Here's how the part is built. I have some questions about the finished solid (model axes, mm). A direction names the side the tool comes from. Give positions to 0.01 mm unless a question says otherwise; leave off trailing zeros. Loops run counter-clockwise (first coordinate to the right, second up) from the corner with the lowest first, then second, coordinate; pieces in that order, holes last. Notation, with made-up numbers: (57, 72.5) - (75, 72.5) arc R25 ccw to (75, 106.5) - close; hole circle Ø5 at (-12.5, 80). An arc over 180 degrees is marked (long way). Use one line per item in the form item = value.
from build123d import *

# Parameters (mm, degrees)
F0_W      = 139.7
F0_H      = 215.9
F1_DEPTH  = 74.7
F2_R      = 17.526
F2_R_2    = 14.351
F2_R_3    = 11.176
F3_DEPTH  = 0.5
F4_R      = 17.526
F4_R_2    = 14.351
F4_R_3    = 11.176
F5_DEPTH  = 1
F4_R_4    = 3.55
F6_DEPTH  = 25
F7_W      = 17.25
F7_H      = 1.4
F8_DEPTH  = 51.1
F10_DEPTH = 139.701
F11_R     = 2


with BuildPart() as f1:
    # F0 (on Right) → F1 (new body, symmetric)
    with BuildSketch(Plane.YZ):
        with Locations((69.85, 107.95)):
            Rectangle(F0_W, F0_H)
    extrude(amount=F1_DEPTH, both=True)

    # F2 (on face) → F3 (cut)
    with BuildSketch(Plane.YZ.offset(74.7)):
        with Locations((88.9, 38.1)):
            Circle(F2_R)
        with Locations((88.9, 38.1)):
            Circle(F2_R_2, mode=Mode.SUBTRACT)
        with Locations((88.9, 38.1)):
            Circle(F2_R_3)
    extrude(amount=-F3_DEPTH, mode=Mode.SUBTRACT)

    # F4 (on face) → F5 (cut)
    with BuildSketch(Plane(origin=(0, 139.7, 0), x_dir=(-1, 0, 0), z_dir=(0, 1, 0))):
        with Locations((42.9, 38.1)):
            Circle(F4_R)
        with Locations((42.9, 38.1)):
            Circle(F4_R_2, mode=Mode.SUBTRACT)
        with Locations((42.9, 38.1)):
            Circle(F4_R_3)
    extrude(amount=-F5_DEPTH, mode=Mode.SUBTRACT)

    # F4 (on face) → F6 (cut)
    with BuildSketch(Plane(origin=(0, 139.7, 0), x_dir=(-1, 0, 0), z_dir=(0, 1, 0))):
        with Locations((0, 31.8)):
            Circle(F4_R_4)
    extrude(amount=-F6_DEPTH, mode=Mode.SUBTRACT)

    # F7 (on face) → F8 (join)
    with BuildSketch(Plane.XY.offset(215.9)):
        with Locations((61.075, 139)):
            Rectangle(F7_W, F7_H)
        with Locations((-61.075, 139)):
            Rectangle(F7_W, F7_H)
    extrude(amount=F8_DEPTH)

    # F9 (on face) → F10 (cut, through all)
    with BuildSketch(Plane(origin=(0, 139.7, 0), x_dir=(-1, 0, 0), z_dir=(0, 1, 0))):
        with BuildLine():
            ThreePointArc((-57.812835, 239.999722), (-57.597703, 240.685223), (-57.525, 241.4))
            ThreePointArc((-57.525, 241.4), (-61.789777, 244.877297), (-64.337165, 239.999722))
            ThreePointArc((-64.337165, 239.999722), (-61.075, 241.4), (-57.812835, 239.999722))
        make_face()
        with BuildLine():
            ThreePointArc((-57.812835, 239.999722), (-61.075, 241.4), (-64.337165, 239.999722))
            ThreePointArc((-64.337165, 239.999722), (-61.075, 237.85), (-57.812835, 239.999722))
        make_face()
        with BuildLine():
            ThreePointArc((-57.812835, 239.999722), (-61.075, 237.85), (-64.337165, 239.999722))
            ThreePointArc((-64.337165, 239.999722), (-62.74387, 232.720901), (-56.575, 236.9))
            ThreePointArc((-56.575, 236.9), (-56.895901, 238.56887), (-57.812835, 239.999722))
        make_face()
        with BuildLine():
            ThreePointArc((64.337165, 239.999722), (64.552297, 240.685223), (64.625, 241.4))
            ThreePointArc((64.625, 241.4), (60.360223, 244.877297), (57.812835, 239.999722))
            ThreePointArc((57.812835, 239.999722), (61.075, 241.4), (64.337165, 239.999722))
        make_face()
        with BuildLine():
            ThreePointArc((64.337165, 239.999722), (61.075, 241.4), (57.812835, 239.999722))
            ThreePointArc((57.812835, 239.999722), (61.075, 237.85), (64.337165, 239.999722))
        make_face()
        with BuildLine():
            ThreePointArc((64.337165, 239.999722), (61.075, 237.85), (57.812835, 239.999722))
            ThreePointArc((57.812835, 239.999722), (59.40613, 232.720901), (65.575, 236.9))
            ThreePointArc((65.575, 236.9), (65.254099, 238.56887), (64.337165, 239.999722))
        make_face()
    extrude(amount=-F10_DEPTH, mode=Mode.SUBTRACT)

    # F11
    f11_edges = [f1.edges().sort_by_distance(p)[0] for p in [
        (-52.45, 139, 267),
        (-69.7, 139, 267),
        (69.7, 139, 267),
        (52.45, 139, 267),
    ]]
    fillet(f11_edges, radius=F11_R)


solid = f1.part
(1) For P1, Ø11, axis at y = 91.5, z = 42.5, coming from the +X side; P2, Ø6.5, axis at x = 61.075, z = 241.4, coming from the -Y side; P3, Ø11.5, axis at x = 61.075, z = 236.9, coming from the -Y side; P4, Ø18, axis at x = -43.5, z = 39.5, coming from the +Y side, each with a flat end and sliding along its axis, tell me the tip position at first contact or that it passes through.
Geometry says:
P1 = 74.2
P2 = through
P3 = 138.3
P4 = 138.7
(2) Thinking about a two-plate mould opening in Y: for faces 1 (the flat face through (-50, 139.7, 47)), 2 (the flat face through (1, 0, 106)), 3 (the cylindrical face through (74.45, 105.62, 43.36)), which applies, pulls with the +Y half, pulls with the -Y half, needs draft (parallel to the pull), parting line crosses it, or undercut?
Geometry says:
face_1 = pulls with the +Y half
face_2 = pulls with the -Y half
face_3 = undercut
(3) If we section it at D-D (y = 17): List the corners of the cut face in (x, z) for me.
Geometry says:
outline = (-74.7, 0) - (74.7, 0) - (74.7, 215.9) - (-74.7, 215.9) - close
(4) If we section it at C-C (x = 0): List the corners of the cut face in (y, z) for me, plus the area to 3 significant figures.
Geometry says:
outline = (0, 0) - (139.7, 0) - (139.7, 28.25) - (114.7, 28.25) - (114.7, 35.35) - (139.7, 35.35) - (139.7, 215.9) - (0, 215.9) - close
area = 30,000 mm²
(5) If I drill on probe 1 along Z at (x, y) = (-42, 139); probe 2 along X at (y, z) = (139, 241); probe 3 along Z at (x, y) = (0, 124), over which ranges is the centre line in solid material (lowest first)?
Geometry says:
probe_1 = 0 to 20.6, 23.78 to 26.96, 49.24 to 52.42, 55.6 to 215.9
probe_2 = -69.7 to -64.6, -57.55 to -52.45, 52.45 to 57.55, 64.6 to 69.7
probe_3 = 0 to 28.25, 35.35 to 215.9
(6) If we section it at A-A (z = 221): List the corners of the cut face in (x, y) for me.
Geometry says:
outline = (-69.7, 138.3) - (-52.45, 138.3) - (-52.45, 139.7) - (-69.7, 139.7) - close; (52.45, 138.3) - (69.7, 138.3) - (69.7, 139.7) - (52.45, 139.7) - close
(7) If we section it at B-B (y = 88.9): List the corners of the cut face in (x, z) for me, plus the area to 3 significant figures.
Geometry says:
outline = (-74.7, 0) - (74.7, 0) - (74.7, 20.57) - (74.2, 20.57) - (74.2, 23.75) - (74.7, 23.75) - (74.7, 26.92) - (74.2, 26.92) - (74.2, 49.28) - (74.7, 49.28) - (74.7, 52.45) - (74.2, 52.45) - (74.2, 55.63) - (74.7, 55.63) - (74.7, 215.9) - (-74.7, 215.9) - close
area = 32,200 mm²
(8) For faces 4 (the flat face through (-57, 138.3, 241)), 5 (the cylindrical face through (74.45, 99.56, 41.46)), 6 (the cylindrical face through (-29.98, 139.21, 49.94)), which set-ups out of +Z, -Z, +X, -X, +Y, -Y let a thin tool reach every point of the face, with its end or its side?
Geometry says:
face_4 = +Z, +X, -X, -Y
face_5 = +X
face_6 = +Y
